Here's how the part is built. I have some questions about the finished solid (model axes, mm). Coordinates: 2 decimals unless noted, no trailing zeros. Loops run counter-clockwise (first coordinate to the right, second up) from the corner with the lowest first, then second, coordinate; pieces in that order, holes last. Notation, with made-up numbers: (32, -33) -> (50, -33) arc R34 ccw to (50, -2) -> close; hole circle Ø3 at (-20.5, 62.5). An arc over 180 degrees is marked (long way). Answer as a JSON object with one key per item and string values. Group by question number.
1) I need wall thicknesses on probe 1 along X at (y, z) = (9.25, 429.5); probe 2 along Y at (x, z) = (-0.5, 221.5); probe 3 along Y at (x, z) = (-5.45, 495.3). Which ranges of each line are inside material? Lowest first, please. Write a range as [from, to].
2) I want a section at A-A (z = 111.5). Write out the boundary of the cut face in (x, y), then the cut area to 3 significant figures.
3) I'm going to push a flat-ended pin straight in: pin 1 (3.5 mm diameter, centred on y = 0, z = 495.3, fed in from +X). Where does the tip first touch, or does it pass through?
4) I want a section at B-B (x = 0). Write out the boundary of the cut face in (y, z).
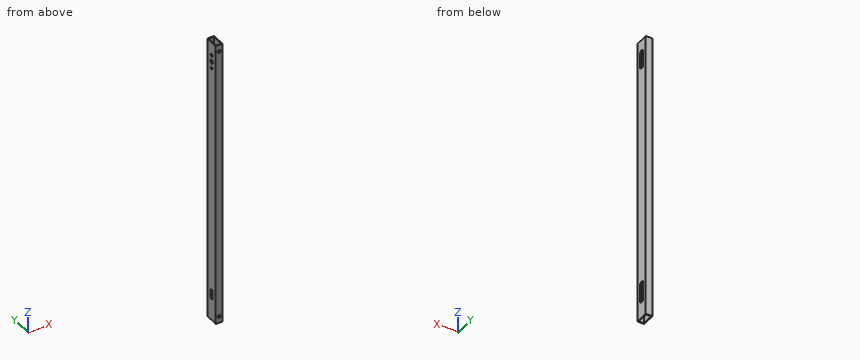
```python
from build123d import *

# Parameters (mm, degrees)
SKETCH1_W           = 12.7
SKETCH1_H           = 25.4
SKETCH1_W_2         = 9.525
SKETCH1_H_2         = 22.225
BOSS_EXTRUDE1_DEPTH = 546.1
SKETCH2_R           = 3.81
SKETCH2_R_2         = 2.75
CUT_EXTRUDE1_DEPTH  = 547.395269013
CUT_EXTRUDE3_REACH  = 548.395
CUT_EXTRUDE5_REACH  = 548.727
SKETCH5_R           = 2.75


with BuildPart() as part:
    # Sketch1 → Boss-Extrude1 (new body)
    with BuildSketch(Plane.XY):
        Rectangle(SKETCH1_W, SKETCH1_H)
        Rectangle(SKETCH1_W_2, SKETCH1_H_2, mode=Mode.SUBTRACT)
    extrude(amount=BOSS_EXTRUDE1_DEPTH)

    # Sketch2 → Cut-Extrude1 (cut, through all)
    with BuildSketch(Plane(origin=(6.35, 0, 0), x_dir=(0, 0, -1), z_dir=(1, 0, 0))):
        with Locations((-508, 0)):
            Circle(SKETCH2_R)
        with Locations((-520.7, 0)):
            Circle(SKETCH2_R_2)
        with Locations((-495.3, 0)):
            Circle(SKETCH2_R_2)
        with BuildLine():
            Line((-44.45, -3.302), (-57.15, -3.302))
            ThreePointArc((-57.15, -3.302), (-60.452, 0), (-57.15, 3.302))
            Line((-57.15, 3.302), (-44.45, 3.302))
            ThreePointArc((-44.45, 3.302), (-41.148, 0), (-44.45, -3.302))
        make_face()
    extrude(amount=-CUT_EXTRUDE1_DEPTH, mode=Mode.SUBTRACT)

    # Sketch4 → Cut-Extrude3 (cut, up to next)
    with BuildSketch(Plane.ZY.offset(-6.35), mode=Mode.PRIVATE) as cut_extrude3_sk1:
        with BuildLine():
            Line((35.56, 5), (66.04, 5))
            ThreePointArc((66.04, 5), (71.04, 0), (66.04, -5))
            Line((66.04, -5), (35.56, -5))
            ThreePointArc((35.56, -5), (30.56, 0), (35.56, 5))
        make_face()
    cut_extrude3_tool1 = extrude(cut_extrude3_sk1.sketch, amount=CUT_EXTRUDE3_REACH, mode=Mode.PRIVATE) & part.part
    # Sketch4 → Cut-Extrude3 (cut, up to next)
    with BuildSketch(Plane.ZY.offset(-6.35), mode=Mode.PRIVATE) as cut_extrude3_sk2:
        with BuildLine():
            Line((495.3, 5), (520.7, 5))
            ThreePointArc((520.7, 5), (525.7, 0), (520.7, -5))
            Line((520.7, -5), (495.3, -5))
            ThreePointArc((495.3, -5), (490.3, 0), (495.3, 5))
        make_face()
    cut_extrude3_tool2 = extrude(cut_extrude3_sk2.sketch, amount=CUT_EXTRUDE3_REACH, mode=Mode.PRIVATE) & part.part
    add(cut_extrude3_tool1.solids().sort_by_distance((6.35, 0, 50.8))[0], mode=Mode.SUBTRACT)
    add(cut_extrude3_tool2.solids().sort_by_distance((6.35, 0, 508))[0], mode=Mode.SUBTRACT)

    # Sketch5 → Cut-Extrude5 (cut, up to next)
    with BuildSketch(Plane.XZ.offset(12.7), mode=Mode.PRIVATE) as cut_extrude5_sk1:
        with Locations(Location((0, 533.4, 0), (0, 0, 270))):
            Circle(SKETCH5_R)
    cut_extrude5_tool1 = extrude(cut_extrude5_sk1.sketch, amount=-CUT_EXTRUDE5_REACH, mode=Mode.PRIVATE) & part.part
    # Sketch5 → Cut-Extrude5 (cut, up to next)
    with BuildSketch(Plane.XZ.offset(12.7), mode=Mode.PRIVATE) as cut_extrude5_sk2:
        with Locations(Location((0, 12.7, 0), (0, 0, 270))):
            Circle(SKETCH5_R)
    cut_extrude5_tool2 = extrude(cut_extrude5_sk2.sketch, amount=-CUT_EXTRUDE5_REACH, mode=Mode.PRIVATE) & part.part
    add(cut_extrude5_tool1.solids().sort_by_distance((0, -12.7, 533.4))[0], mode=Mode.SUBTRACT)
    add(cut_extrude5_tool2.solids().sort_by_distance((0, -12.7, 12.7))[0], mode=Mode.SUBTRACT)


solid = part.part
```
Determined:
{
 "1": {"probe 1": "[-6.35, -4.76], [4.76, 6.35]", "probe 2": "[-12.7, -11.11], [11.11, 12.7]", "probe 3": "[-12.7, -2.75], [2.75, 12.7]"},
 "2": {"outline": "(-6.35, -12.7) -> (6.35, -12.7) -> (6.35, 12.7) -> (-6.35, 12.7) -> close; hole (-4.76, -11.11) -> (4.76, -11.11) -> (4.76, 11.11) -> (-4.76, 11.11) -> close", "area": "111 mm^2"},
 "3": {"pin 1": "through"},
 "4": {"outline": "(-12.7, 0) -> (-11.11, 0) -> (-11.11, 9.95) -> (-12.7, 9.95) -> close; (-12.7, 15.45) -> (-11.11, 15.45) -> (-11.11, 530.65) -> (-12.7, 530.65) -> close; (-12.7, 536.15) -> (-11.11, 536.15) -> (-11.11, 546.1) -> (-12.7, 546.1) -> close; (11.11, 0) -> (12.7, 0) -> (12.7, 546.1) -> (11.11, 546.1) -> close"}
}
